from build123d import *

# Parameters (mm, degrees)
SKETCH1_W           = 177.8
SKETCH1_H           = 63.5
BOSS_EXTRUDE1_DEPTH = 45.72
SKETCH2_W           = 101.6
SKETCH2_H           = 63.5
CUT_EXTRUDE1_DEPTH  = 9.525
SKETCH3_W           = 166.116
SKETCH3_H           = 54.864
CUT_EXTRUDE2_DEPTH  = 42.545
SKETCH4_R           = 6.096
CUT_EXTRUDE3_DEPTH  = 31.75
CUT_EXTRUDE4_START  = -43.18
SKETCH5_R           = 4.445
CUT_EXTRUDE4_DEPTH  = 31.75
SKETCH9_W           = 6.35
SKETCH9_H           = 6.35
SKETCH9_W_2         = 6.565288585
SKETCH9_W_3         = 7.62
SKETCH9_H_2         = 7.62
BOSS_EXTRUDE2_DEPTH = 10.16
BOSS_EXTRUDE2_TAPER = 14
SKETCH6_W           = 56.642
SKETCH6_H           = 43.307
CUT_EXTRUDE5_DEPTH  = 33.02
SKETCH8_R           = 1.5875
CUT_EXTRUDE7_DEPTH  = 4.572
FILLET1_R           = 1.27
FILLET2_R           = 1.27
SKETCH10_W          = 6.35
SKETCH10_H          = 6.604
SKETCH10_W_2        = 7.62
SKETCH10_H_2        = 7.62
BOSS_EXTRUDE3_DEPTH = 10.16
BOSS_EXTRUDE3_TAPER = 13
SKETCH7_R           = 1.5875
CUT_EXTRUDE6_DEPTH  = 4.572
FILLET3_R           = 1.27


with BuildPart() as part:
    # Sketch1 → Boss-Extrude1 (new body)
    with BuildSketch(Plane.XY):
        Rectangle(SKETCH1_W, SKETCH1_H)
    extrude(amount=BOSS_EXTRUDE1_DEPTH)

    # Sketch2 → Cut-Extrude1 (cut)
    with BuildSketch(Plane.XY.offset(45.72)):
        with Locations((-38.1, 0)):
            Rectangle(SKETCH2_W, SKETCH2_H)
    extrude(amount=-CUT_EXTRUDE1_DEPTH, mode=Mode.SUBTRACT)

    # Sketch3 → Cut-Extrude2 (cut)
    with BuildSketch(Plane.XY.offset(45.72)):
        Rectangle(SKETCH3_W, SKETCH3_H)
    extrude(amount=-CUT_EXTRUDE2_DEPTH, mode=Mode.SUBTRACT)

    # Sketch4 → Cut-Extrude3 (cut)
    with BuildSketch(Plane(origin=(88.9, 0, 0), x_dir=(0, 0, -1), z_dir=(1, 0, 0))):
        with Locations((-15.24, 0)):
            Circle(SKETCH4_R)
    extrude(amount=-CUT_EXTRUDE3_DEPTH, mode=Mode.SUBTRACT)

    # Sketch5 → Cut-Extrude4 (cut)
    with BuildSketch(Plane(origin=(0, 31.75, 0), x_dir=(1, 0, 0), z_dir=(0, 1, 0)).offset(CUT_EXTRUDE4_START)):
        with Locations(Location((46.900902689, -35.56, 0), (0, 0, 180))):  # turned: the seam where the file's is
            Circle(SKETCH5_R)
    extrude(amount=-CUT_EXTRUDE4_DEPTH, mode=Mode.SUBTRACT)

    # Sketch9 → Boss-Extrude2 (add)
    with BuildSketch(Plane.XY.offset(36.195)):
        with Locations((5.78513156, 28.575)):
            Rectangle(SKETCH9_W, SKETCH9_H)
        with Locations((-28.41302197, 28.575)):
            Rectangle(SKETCH9_W_2, SKETCH9_H)
        with Locations((5.78513156, -28.575)):
            Rectangle(SKETCH9_W, SKETCH9_H)
        with Locations((-85.09, -27.94)):
            Rectangle(SKETCH9_W_3, SKETCH9_H_2)
    extrude(amount=-BOSS_EXTRUDE2_DEPTH, taper=BOSS_EXTRUDE2_TAPER)

    # Sketch6 → Cut-Extrude5 (cut)
    with BuildSketch(Plane.XY.offset(36.195)):
        with Locations((-60.579, 10.0965)):
            Rectangle(SKETCH6_W, SKETCH6_H)
    extrude(amount=-CUT_EXTRUDE5_DEPTH, mode=Mode.SUBTRACT)

    # Sketch8 → Cut-Extrude7 (cut)
    with BuildSketch(Plane.XY.offset(36.195)):
        with Locations((5.996300657, 28.702)):
            Circle(SKETCH8_R)
        with Locations((-28.340687554, 28.702)):
            Circle(SKETCH8_R)
        with Locations((5.996300657, -28.702)):
            Circle(SKETCH8_R)
        with Locations((-85.09, -27.94)):
            Circle(SKETCH8_R)
    extrude(amount=-CUT_EXTRUDE7_DEPTH, mode=Mode.SUBTRACT)

    # Fillet1
    fillet1_edges = [part.edges().sort_by_distance(p)[0] for p in [
        (-32.258, 31.75, 19.685),
        (-88.9, -31.75, 18.0975),
        (88.9, 31.75, 22.86),
        (88.9, -31.75, 22.86),
    ]]
    fillet(fillet1_edges, radius=FILLET1_R)

    # Fillet2
    fillet2_edges = [part.edges().sort_by_distance(p)[0] for p in [
        (-88.9, -11.557, 19.685),
    ]]
    fillet(fillet2_edges, radius=FILLET2_R)

    # Sketch10 → Boss-Extrude3 (add)
    with BuildSketch(Plane.XY.offset(45.72)):
        with Locations((19.538431576, 28.448)):
            Rectangle(SKETCH10_W, SKETCH10_H)
        with Locations((84.718025612, 27.568025612)):
            Rectangle(SKETCH10_W_2, SKETCH10_H_2)
        with Locations((84.718025612, -27.568025612)):
            Rectangle(SKETCH10_W_2, SKETCH10_H_2)
        with Locations((19.538431576, -28.448)):
            Rectangle(SKETCH10_W, SKETCH10_H)
    extrude(amount=-BOSS_EXTRUDE3_DEPTH, taper=BOSS_EXTRUDE3_TAPER)

    # Sketch7 → Cut-Extrude6 (cut)
    with BuildSketch(Plane.XY.offset(45.72)):
        with Locations((85.344, 28.194)):
            Circle(SKETCH7_R)
        with Locations(Location((85.344, -28.194, 0), (0, 0, 180))):  # turned: the seam where the file's is
            Circle(SKETCH7_R)
        with Locations((19.538431576, 28.194)):
            Circle(SKETCH7_R)
        with Locations((19.538431576, -28.194)):
            Circle(SKETCH7_R)
    extrude(amount=-CUT_EXTRUDE6_DEPTH, mode=Mode.SUBTRACT)

    # Fillet3
    fillet3_edges = [part.edges().sort_by_distance(p)[0] for p in [
        (-88.9, 31.75, 1.5875),
    ]]
    fillet(fillet3_edges, radius=FILLET3_R)


solid = part.part
Can you work these out from the model? Positions are in its coordinate system, mm. A direction names the side the tool comes from. Round coordinates to 2 decimals unless told otherwise and drop trailing zeros. Write each loop counter-clockwise with the first axis right and the second up, starting at its lowest first coordinate (ties: lowest second). Pieces come first, ordered by that corner, then holes. Notation, with made-up numbers: (68, -4) -> (84, -4) arc R3 ccw to (84, 0) -> close; hole circle Ø1 at (45.25, -23). An arc over 180 degrees is marked (long way). One line per question, with ' | ' between items. Start each with the question number.
1) Suppose I cut it at D-D on x = 35. Write out the boundary of the cut face in (y, z) (3 decimals), then the cut area to 3 significant figures.
2) I'm going to push flat-ended pins straight in: P1, Ø3.5, axis at y = 29, z = 27, coming from the -X side; P2, Ø5, axis at x = -8.5, y = 27, coming from the +Z side (3 decimals); P3, Ø11.5, axis at x = 46.9, z = 35.56, coming from the -Y side; P4, Ø4.5, axis at y = -29, z = 42, coming from the -X side. Where does each tip first touch, or does it pass through?
3) Suppose I cut it at B-B on y = 0. Write out the boundary of the cut face in (x, z) (3 decimals), then the cut area to 3 significant figures.
4) Suppose I cut it at A-A on z = 15.24. Write out the boundary of the cut face in (x, y).
5) I need wall thicknesses on line 1 (Y direction, x = 31, z = 20.5); line 2 (X direction, y = -14.5, z = 15); line 3 (Z direction, x = 19.5, y = -0.5) (3 decimals). Which ranges of each line are inside material? Lowest first, please. Write a range as [from, to].
6) If we mould it in two halves opening along Y, with no side actions, what happens to faces 1 (the flat face through (85, 28, 41.148)), 2 (the flat face through (-85, -11.557, 20)), 3 (the flat face through (-11, 30, 36.195))? For each: released by +Y, released by -Y, zero draft, split by the parting line, or undercut.
7) On a 3-axis mill with a long thin cutter (end or side, diameter ignored), from which of +Z, -Z, +X, -X, +Y, -Y can I reach the whole of each face in a straight line? I mean faces 4 (the flat face through (20, 28, 41.148)), 5 (the flat face through (12.7, -30, 41)), 6 (the flat face through (-83.058, -20, 20)), 7 (the flat face through (83.5, 3.2, 45.72)). Say none if no direction works.
8) Suppose I cut it at C-C on y = 11.5. Write out the boundary of the cut face in (x, z) (3 decimals), then the cut area to 3 significant figures.
Return value:
1) outline: (-31.75, 0) -> (31.75, 0) -> (31.75, 45.72) -> (27.432, 45.72) -> (27.432, 3.175) -> (-27.432, 3.175) -> (-27.432, 45.72) -> (-31.75, 45.72) -> close | area: 569 mm2
2) P1: stops at x = -32.26 | P2: stops at z = 36.195 | P3: stops at y = -31.75 | P4: stops at x = 12.7
3) outline: (-88.9, 0) -> (88.9, 0) -> (88.9, 9.144) -> (83.058, 9.144) -> (83.058, 3.175) -> (-88.9, 3.175) -> close; (83.058, 21.336) -> (88.9, 21.336) -> (88.9, 45.72) -> (83.058, 45.72) -> close | area: 742 mm2
4) outline: (-88.9, -30.48) arc R1.27 ccw to (-87.63, -31.75) -> (87.63, -31.75) arc R1.27 ccw to (88.9, -30.48) -> (88.9, -6.1) -> (83.06, -6.1) -> (83.06, -27.43) -> (-83.06, -27.43) -> (-83.06, -11.56) -> (-87.63, -11.56) arc R1.27 ccw to (-88.9, -12.83) -> close; (-32.26, 27.43) -> (83.06, 27.43) -> (83.06, 6.1) -> (88.9, 6.1) -> (88.9, 30.48) arc R1.27 ccw to (87.63, 31.75) -> (-30.99, 31.75) arc R1.27 ccw to (-32.26, 30.48) -> close
5) line 1: y = [-31.75, -27.43], [27.43, 31.75] | line 2: x = [-88.9, -83.06], [83.06, 88.9] | line 3: z = [0, 3.175]
6) face 1: undercut | face 2: released by +Y | face 3: zero draft
7) face 4: +Z | face 5: +Z, -X, +Y, -Y | face 6: +Y | face 7: +Z, +X, -X, +Y, -Y
8) outline: (-88.9, 0) -> (88.9, 0) -> (88.9, 45.72) -> (83.058, 45.72) -> (83.058, 3.175) -> (-88.9, 3.175) -> close | area: 813 mm2
